Build history of the part. All positions in model axes, mm. Coordinates: 2 decimals unless noted, no trailing zeros. Loops run counter-clockwise (first coordinate to the right, second up) from the corner with the lowest first, then second, coordinate; pieces in that order, holes last.
(1) Wall check: L1, parallel to Z at x = 0, y = -4.5; L2, parallel to X at y = -13.25, z = 27; L3, parallel to X at y = -6.75, z = 25 (3 decimals). Give the ranges that are in metal, low to high.
(2) Slice it at C-C (y = -9). Give the cut face in (x, z), and give its area (3 significant figures).
(3) Slice it at A-A (x = 0). Give the cut face in (y, z).
(4) Flat gauge pins, fed straight in: P1, Ø4, axis at x = 0, z = 41, coming from the +Y side; P2, Ø2, axis at y = -8, z = -32.5, coming from the -X side; P3, Ø2, axis at y = -15, z = -1, coming from the -X side. Where does each tip first touch, or does it go through?
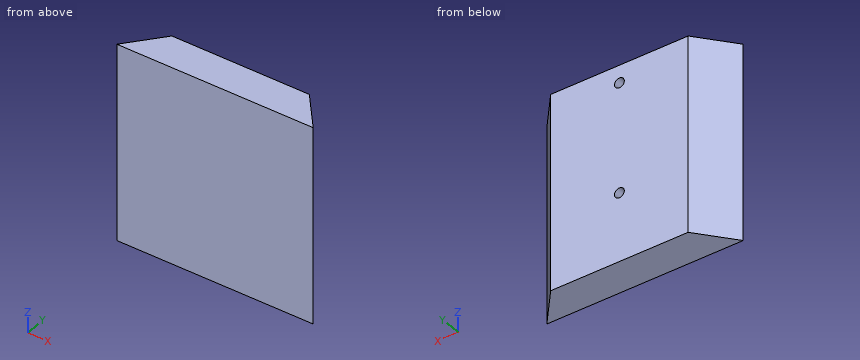
from build123d import *

# Parameters (mm, degrees)
F0_W       = 100
F0_H       = 100
F1_DEPTH   = 18
F2_SIZE2   = 14.99999
F2_SIZE    = 17.99999
F2_2_SIZE2 = 14.99999
F2_2_SIZE  = 17.99999
F3_R       = 2.5
F4_DEPTH   = 15


# Not quite as in the source:
# - a fillet or chamfer is up to 0.001 mm smaller than in the source, because OpenCascade refuses the exact size


with BuildPart() as f1:
    # F0 (on Front) → F1 (new body)
    with BuildSketch(Plane.XZ):
        Rectangle(F0_W, F0_H)
    extrude(amount=F1_DEPTH)

    # F2 (size 18 and 15 in the source; OpenCascade refuses exactly that, so slightly less here)
    f2_edges = [f1.edges().sort_by_distance(p)[0] for p in [
        (50, 0, 0),
    ]]
    f2_side = f1.faces().sort_by_distance((50, -9, 0))[0]
    chamfer(f2_edges, length=F2_SIZE, length2=F2_SIZE2, reference=f2_side)

    # F2#2 (size 18 and 15 in the source; OpenCascade refuses exactly that, so slightly less here)
    f2_2_edges = [f1.edges().sort_by_distance(p)[0] for p in [
        (-50, 0, 0),
    ]]
    f2_2_side = f1.faces().sort_by_distance((-50, -9, 0))[0]
    chamfer(f2_2_edges, length=F2_2_SIZE, length2=F2_2_SIZE2, reference=f2_2_side)

    # F3 (on face) → F4 (cut)
    with BuildSketch(Plane(origin=(0, 0, 0), x_dir=(-1, 0, 0), z_dir=(0, 1, 0))):
        with Locations((0, -15)):
            Circle(F3_R)
        with Locations((0, 41)):
            Circle(F3_R)
    extrude(amount=-F4_DEPTH, mode=Mode.SUBTRACT)


solid = f1.part
Response values:
1. L1: z = -50 to -17.5, -12.5 to 38.5, 43.5 to 50
1. L2: x = -46.04 to 46.04
1. L3: x = -40.625 to 40.625
2. outline: (-42.5, -50) - (42.5, -50) - (42.5, 50) - (-42.5, 50) - close; hole circle Ø5 at (0, -15); hole circle Ø5 at (0, 41)
2. area: 8,460 mm2
3. outline: (-18, -50) - (0, -50) - (0, -17.5) - (-15, -17.5) - (-15, -12.5) - (0, -12.5) - (0, 38.5) - (-15, 38.5) - (-15, 43.5) - (0, 43.5) - (0, 50) - (-18, 50) - close
4. P1: stops at y = -15
4. P2: stops at x = -42.5
4. P3: stops at x = -48.33
